Build history of the part. All positions in model axes, mm. A direction names the side the tool comes from. Round coordinates to 2 decimals unless told otherwise and drop trailing zeros. Loops run counter-clockwise (first coordinate to the right, second up) from the corner with the lowest first, then second, coordinate; pieces in that order, holes last. Notation, with made-up numbers: (-8.5, 2) - (4.5, 2) arc R16 cw to (4.5, 24) - close; hole circle Ø11 at (29, -6.75). An arc over 180 degrees is marked (long way). Use a Markdown table: item, result.
from build123d import *

# Parameters (mm, degrees)
SKETCH1_R           = 1.5
SKETCH1_W           = 20
SKETCH1_H           = 3.2
BOSS_EXTRUDE1_DEPTH = 3


with BuildPart() as part:
    # Sketch1 → Boss-Extrude1 (new body)
    with BuildSketch(Plane.XY):
        Polygon((10, -48), (-10, -48), (-10, -45), (-35, -45), (-35, 0), (-58, 0), (-58, 53), (-10, 53), (-10, 56), (10, 56), (10, 53), (58, 53), (58, 0), (35, 0), (35, -45), (10, -45), align=None)
        with Locations((-30, 0)):
            Circle(SKETCH1_R, mode=Mode.SUBTRACT)
        with Locations((-30, -35)):
            Circle(SKETCH1_R, mode=Mode.SUBTRACT)
        with Locations((30, 0)):
            Circle(SKETCH1_R, mode=Mode.SUBTRACT)
        with Locations((30, -35)):
            Circle(SKETCH1_R, mode=Mode.SUBTRACT)
        with Locations((-30, 11)):
            Circle(SKETCH1_R, mode=Mode.SUBTRACT)
        with Locations((-30, 46)):
            Circle(SKETCH1_R, mode=Mode.SUBTRACT)
        with Locations((30, 46)):
            Circle(SKETCH1_R, mode=Mode.SUBTRACT)
        with Locations((30, 11)):
            Circle(SKETCH1_R, mode=Mode.SUBTRACT)
        with Locations((0, 1.6)):
            Rectangle(SKETCH1_W, SKETCH1_H, mode=Mode.SUBTRACT)
    extrude(amount=BOSS_EXTRUDE1_DEPTH)


solid = part.part
Q1. Which spindle directions (+Z, -Z, +X, -X, +Y, -Y) get a long thin tool onto all of the face, cutting with end or side? Do faces 4 (the face through (-46, 0, 1)), 5 (the face through (0, 3.2, 1)), 6 (the face through (-34, 53, 1)). Say none if no direction does.
Results found:
| item | result |
|---|---|
| face 4 | +Z, -Z, -X, -Y |
| face 5 | +Z, -Z |
| face 6 | +Z, -Z, -X, +Y |
Q2. Cut at D-D, the plane x = 30. List the corners of the cut face in (y, z), plus the area to 3 significant figures.
Results found:
| item | result |
|---|---|
| outline | (-45, 0) - (-36.5, 0) - (-36.5, 3) - (-45, 3) - close; (-33.5, 0) - (-1.5, 0) - (-1.5, 3) - (-33.5, 3) - close; (1.5, 0) - (9.5, 0) - (9.5, 3) - (1.5, 3) - close; (12.5, 0) - (44.5, 0) - (44.5, 3) - (12.5, 3) - close; (47.5, 0) - (53, 0) - (53, 3) - (47.5, 3) - close |
| area | 258 mm2 |
Q3. Drop flat-ended pins along their axis: pin 1 (0.9 mm diameter, centred on y = -21.5, z = 1, fed in from +X); pin 2 (1.5 mm diameter, centred on x = -16.5, z = 1.5, fed in from -Y); pin 3 (0.9 mm diameter, centred on x = -50.5, z = 1.5, fed in from -Y). Give the stop position or say it passes through.
Results found:
| item | result |
|---|---|
| pin 1 | stops at x = 35 |
| pin 2 | stops at y = -45 |
| pin 3 | stops at y = 0 |
Q4. Pull direction Y, two halves, no side cores. Call faces 1 (the face through (-31.5, 0.07, 1.48)), 2 (the face through (0, 56, 1)), 3 (the face through (-10, 54, 1)): pulls with the +Y half, pulls with the -Y half, needs draft (parallel to the pull), parting line crosses it, or undercut.
Results found:
| item | result |
|---|---|
| face 1 | undercut |
| face 2 | pulls with the +Y half |
| face 3 | needs draft |
Q5. Cut at C-C, the plane x = 8.5. List the corners of the cut face in (y, z).
Results found:
| item | result |
|---|---|
| outline | (-48, 0) - (0, 0) - (0, 3) - (-48, 3) - close; (3.2, 0) - (56, 0) - (56, 3) - (3.2, 3) - close |
Q6. Cut at B-B, the plane z = 0.5. Count the separate pieces of the cut face and the enclosed holes in it, plus the area to 3 significant figures.
Results found:
| item | result |
|---|---|
| separate pieces | 1 |
| enclosed holes | 9 |
| area | 9,300 mm2 |
Q7. Probe line 1 (Y direction, x = 30, z = 2.3); line 2 (Y direction, x = -40.5, z = 2.05); line 3 (X direction, y = 46.5, z = 2.1). List the from-to ranges inside material, lowest first.
Results found:
| item | result |
|---|---|
| line 1 | y = -45 to -36.5, -33.5 to -1.5, 1.5 to 9.5, 12.5 to 44.5, 47.5 to 53 |
| line 2 | y = 0 to 53 |
| line 3 | x = -58 to -31.41, -28.59 to 28.59, 31.41 to 58 |
Q8. Cut at A-A, the plane y = 46. List the corners of the cut face in (x, z), plus the area to 3 significant figures.
Results found:
| item | result |
|---|---|
| outline | (-58, 0) - (-31.5, 0) - (-31.5, 3) - (-58, 3) - close; (-28.5, 0) - (28.5, 0) - (28.5, 3) - (-28.5, 3) - close; (31.5, 0) - (58, 0) - (58, 3) - (31.5, 3) - close |
| area | 330 mm2 |
